The listing builds one solid part. Answer for the finished solid, in the listing's coordinates (mm). Face numbers are marked on the shaded views. A direction names the side the tool comes from. Coordinates: 2 decimals unless noted, no trailing zeros. Loops run counter-clockwise (first coordinate to the right, second up) from the corner with the lowest first, then second, coordinate; pieces in that order, holes last. Notation, with made-up numbers: M -26,-14.75 L 32,-14.75 A26 ccw 32,2.25 Z; hole C 88,47 d6. An arc over 180 degrees is marked long. Answer as a JSON object with one key per item and string values. Group by question number.
1. For the marked faces 4, 5 and 6, determine the directions among +Z, -Z, +X, -X, +Y, -Y from which every point of the face is accessible in a straight line to the end or side of a thin tool.
2. Given pin 1 (5 mm diameter, centred on y = 12.5, z = 39, fed in from -X); pin 2 (2 mm diameter, centred on x = 31.5, y = 17.5, fed in from -Z), each flat-ended and moving along its own axis, determine where each tip first touches the part or whether it passes through.
3. A cutting plane is placed at A-A on z = 37.75. Give the vertices of the cut face in (x, y).
4. A cutting plane is placed at B-B on z = 36. Give the vertices of the cut face in (x, y).
5. A cutting plane is placed at D-D on x = 28.5. Give the vertices of the cut face in (y, z), and give its area (3 significant figures).
6. A cutting plane is placed at C-C on x = 34. Give the vertices of the cut face in (y, z).
7. Determine the mould class of the marked faces 1, 2 and 3 for opening direction Z: released by +Z, released by -Z, zero draft, split by the parting line, or undercut.
8. Straight lines are drawn through the part: L1, parallel to X at y = 19, z = 37; L2, parallel to Z at x = 31, y = 13.75; L3, parallel to X at y = 19.25, z = 35.75. For each, find the intervals that lie inside material, in ascending order.
from build123d import *

# Parameters (mm, degrees)
BOSS_EXTRUDE1_DEPTH      = 7.5
BOSS_EXTRUDE1_DEPTH_BACK = 7.5
FILLET3_R                = 1
FILLET4_R                = 1
FILLET5_R                = 0.5


# Some blends are built 0.0001 mm under size
with BuildPart() as part:
    # Sketch1 → Boss-Extrude1 (new, two sides: drawn at the far end of the back side and taken through both)
    with BuildSketch(Plane.XZ.offset(-16.5).offset(-BOSS_EXTRUDE1_DEPTH_BACK)):
        with BuildLine():
            Line((32.25, 34.5), (32.25, 35.5))
            ThreePointArc((32.25, 35.5), (31.660669064, 36.78109942), (30.471806841, 37.539474849))
            ThreePointArc((30.471806841, 37.539474849), (29.759917895, 38.640489944), (30.75, 39.5))
            Line((30.75, 39.5), (32.75, 39.5))
            ThreePointArc((32.75, 39.5), (33.103553391, 39.353553391), (33.25, 39))
            Line((33.25, 39), (33.25, 31.5))
            Line((33.25, 31.5), (35.25, 31.5))
            Line((35.25, 31.5), (35.25, 39.5))
            ThreePointArc((35.25, 39.5), (34.664213562, 40.914213562), (33.25, 41.5))
            Line((33.25, 41.5), (30.75, 41.5))
            ThreePointArc((30.75, 41.5), (27.781428489, 38.933108746), (29.892857143, 35.625055458))
            ThreePointArc((29.892857143, 35.625055458), (30.150891863, 35.444705186), (30.25, 35.145898034))
            Line((30.25, 35.145898034), (30.25, 34.5))
            ThreePointArc((30.25, 34.5), (29.986067977, 33.381966011), (29.25, 32.5))
            Line((29.25, 32.5), (30.25, 32.5))
            ThreePointArc((30.25, 32.5), (31.664213562, 33.085786438), (32.25, 34.5))
        make_face()
    extrude(amount=BOSS_EXTRUDE1_DEPTH + BOSS_EXTRUDE1_DEPTH_BACK)

    # Fillet3
    # the kernel refuses this fillet: 1 mm, written as the material it takes off along each edge
    with BuildSketch(Plane(origin=(29.25, 5.673991819, 32.5), x_dir=(1, 0, 0), z_dir=(0, 1, 0))) as fillet3_piece_1:
        with BuildLine():
            CenterArc((1.738981007, -0.673726259), FILLET3_R, 137.644685186, 64.623066475)
            ThreePointArc((0.813557862, -1.052661613), (0.478087463, -0.471219443), (0, 0))
            Line((0, 0), (1, 0))
        make_face()
    extrude(amount=21.652016361, mode=Mode.SUBTRACT)

    # Fillet4
    fillet4_edges = [part.edges().sort_by_distance(p)[0] for p in [
        (35.25, 16.5, 31.5),
        (33.25, 16.5, 31.5),
    ]]
    fillet(fillet4_edges, radius=FILLET4_R - 0.0001)  # a hair under: the kernel refuses the full size

    # Fillet5
    fillet5_edges = [part.edges().sort_by_distance(p)[0] for p in [
        (30.25, 16.5, 32.5),
    ]]
    fillet(fillet5_edges, radius=FILLET5_R)


solid = part.part
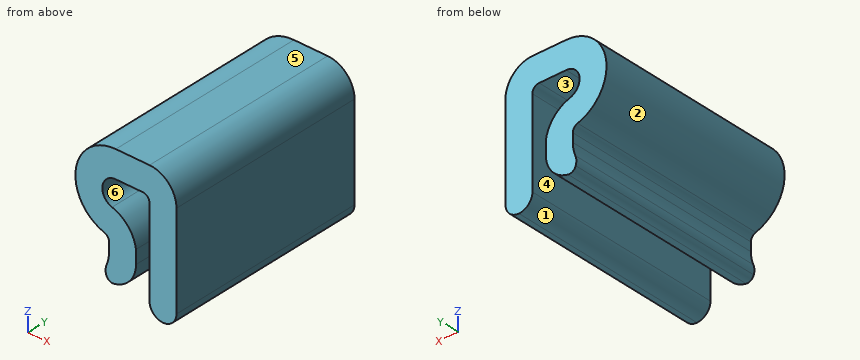
From the geometry:
{
 "1": {"face 4": "-Z, +Y, -Y", "face 5": "+Z, +X, -X, +Y, -Y", "face 6": "+Y, -Y"},
 "2": {"pin 1": "stops at x = 27.75", "pin 2": "stops at z = 32.52"},
 "3": {"outline": "M 27.85,9 L 30.09,9 L 30.09,24 L 27.85,24 Z; M 33.25,9 L 35.25,9 L 35.25,24 L 33.25,24 Z"},
 "4": {"outline": "M 29.09,9 L 32.12,9 L 32.12,24 L 29.09,24 Z; M 33.25,9 L 35.25,9 L 35.25,24 L 33.25,24 Z"},
 "5": {"outline": "M 9,36.52 L 24,36.52 L 24,40.48 L 9,40.48 Z", "area": "59.5 mm²"},
 "6": {"outline": "M 9,31.53 L 24,31.53 L 24,41.35 L 9,41.35 Z"},
 "7": {"face 1": "released by -Z", "face 2": "split by the parting line", "face 3": "undercut"},
 "8": {"L1": "x = 28.15 to 31.44, 33.25 to 35.25", "L2": "z = 32.65 to 37.32, 39.5 to 41.5", "L3": "x = 29.55 to 32.2, 33.25 to 35.25"}
}
